Geometry check sheet. Reference: the model listing, model coordinates, mm. Give positions to 0.01 mm unless a question says otherwise; leave off trailing zeros. Write each loop counter-clockwise with the first axis right and the second up, starting at its lowest first coordinate (ties: lowest second). Pieces come first, ordered by that corner, then holes. Notation, with made-up numbers: M 34.5,89.5 L 69.5,89.5 A27 ccw 69.5,117.5 Z; hole C 4,-0.75 d1. An arc over 180 degrees is marked long. Write each question's results on one line, items separated by ' | '.
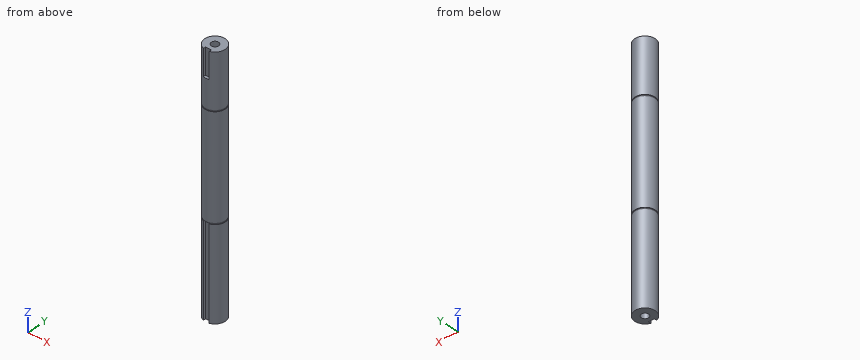
```python
from build123d import *

# Parameters (mm, degrees)
SKETCH_1_R          = 12.5
EXTRUDE_1_DEPTH     = 305.836309
CUT_EXTRUDE_START   = -31.8
SKETCH_2_W          = 7
SKETCH_2_H          = 7
CUT_EXTRUDE_1_DEPTH = 31.8
CUT_EXTRUDE_START_2 = -112
SKETCH_3_W          = 7
SKETCH_3_H          = 7
CUT_EXTRUDE_2_DEPTH = 112
M10X1_251_D         = 8.8
M10X1_251_DEPTH     = 26.25
M10X1_251_TIP       = 2.643786724
M10X1_252_D         = 8.8
M10X1_252_DEPTH     = 26.25
M10X1_252_TIP       = 2.643786724
SKETCH_8_W          = 1.5
SKETCH_8_H          = 0.75


with BuildPart() as part:
    # Эскиз1 → Бобышка-Вытянуть1 (new body)
    with BuildSketch(Plane.XY):
        Circle(SKETCH_1_R)
    extrude(amount=-EXTRUDE_1_DEPTH)

    # Эскиз2 → Вырез-Вытянуть1 (cut)
    with BuildSketch(Plane.XY.offset(CUT_EXTRUDE_START)):
        with Locations((0, -12.5)):
            Rectangle(SKETCH_2_W, SKETCH_2_H)
    extrude(amount=CUT_EXTRUDE_1_DEPTH, mode=Mode.SUBTRACT)

    # Эскиз3 → Вырез-Вытянуть2 (cut)
    with BuildSketch(Plane(origin=(0, 0, -305.836309448), x_dir=(-1, 0, 0), z_dir=(0, 0, -1)).offset(CUT_EXTRUDE_START_2)):
        with Locations((0, -12.5)):
            Rectangle(SKETCH_3_W, SKETCH_3_H)
    extrude(amount=CUT_EXTRUDE_2_DEPTH, mode=Mode.SUBTRACT)

    # Отверстие обработанное метчиком M10x1.251
    with Locations(Plane.XY):
        with Locations((0, 0)):
            Hole(M10X1_251_D / 2, depth=M10X1_251_DEPTH)
            with Locations((0, 0, -(M10X1_251_DEPTH + M10X1_251_TIP / 2))):  # 118° drill point
                Cone(0, M10X1_251_D / 2, M10X1_251_TIP, mode=Mode.SUBTRACT)

    # Отверстие обработанное метчиком M10x1.252
    with Locations(Plane(origin=(0, 0, -305.836309448), x_dir=(-1, 0, 0), z_dir=(0, 0, -1))):
        with Locations((0, 0)):
            Hole(M10X1_252_D / 2, depth=M10X1_252_DEPTH)
            with Locations((0, 0, -(M10X1_252_DEPTH + M10X1_252_TIP / 2))):  # 118° drill point
                Cone(0, M10X1_252_D / 2, M10X1_252_TIP, mode=Mode.SUBTRACT)

    # Эскиз8 → Вырез-Повернуть1 (revolve, cut)
    with BuildSketch(Plane(origin=(0, 0, 0), x_dir=(0, 0, -1), z_dir=(1, 0, 0))):
        with Locations((66.45, 12.125)):
            Rectangle(SKETCH_8_W, SKETCH_8_H)
        with Locations((193.386309448, 12.125)):
            Rectangle(SKETCH_8_W, SKETCH_8_H)
    revolve(axis=Axis((0, 0, 1000), (0, 0, -1)), mode=Mode.SUBTRACT)


solid = part.part
```
Q1. Depth check by flat-ended pin: P1, Ø0.9, axis at y = -10.5, z = -13.5, coming from the +X side; P2, Ø5, axis at y = -4.5, z = -89, coming from the +X side; P3, Ø0.8, axis at x = -1.5, y = -10, coming from the -Z side. Enter the tip coordinate at first touch or a pass-through.
Answer key:
P1: stops at x = 7.43 | P2: stops at x = 12.34 | P3: stops at z = -193.84
Q2. Material ranges on probe 1 along Z at (x, y) = (-4.25, 11); probe 2 along X at (y, z) = (0, -17); probe 3 along Y at (x, z) = (0, -6.25), recorded low to high. Write a range as [from, to].
Answer key:
probe 1: z = [-305.84, -194.14], [-192.64, -67.2], [-65.7, 0] | probe 2: x = [-12.5, -4.4], [4.4, 12.5] | probe 3: y = [-9, -4.4], [4.4, 12.5]
Q3. Section check B-B (z = -182). Enter the section's corners in (x, y).
Answer key:
outline: C 0,0 d25
Q4. Section check A-A (x = -7). Enter the section's corners in (y, z), then the cut area to 3 significant figures.
Answer key:
outline: M -10.36,-305.84 L 10.36,-305.84 L 10.36,-194.14 L 9.44,-194.14 L 9.44,-192.64 L 10.36,-192.64 L 10.36,-67.2 L 9.44,-67.2 L 9.44,-65.7 L 10.36,-65.7 L 10.36,0 L -10.36,0 L -10.36,-65.7 L -9.44,-65.7 L -9.44,-67.2 L -10.36,-67.2 L -10.36,-192.64 L -9.44,-192.64 L -9.44,-194.14 L -10.36,-194.14 Z | area: 6,330 mm2
